from build123d import *

# Parameters (mm, degrees)
EXTRUDE_THIN1_DEPTH = 12.7
CUT_EXTRUDE1_REACH  = 74.956
SKETCH2_R           = 2.25
CUT_EXTRUDE2_REACH  = 74.956
SKETCH6_R           = 1.5


with BuildPart() as part:
    # Sketch1 → Extrude-Thin1 (new body)
    with BuildSketch(Plane.XY):
        Polygon((0, 0), (0, 50.8), (50.8, 50.8), (50.8, 47.625), (3.175, 47.625), (3.175, 0), align=None)
    extrude(amount=EXTRUDE_THIN1_DEPTH)

    # Sketch2 → Cut-Extrude1 (cut, up to next)
    with BuildSketch(Plane.ZY, mode=Mode.PRIVATE) as cut_extrude1_sk1:
        with Locations((6.35, 12.7)):
            Circle(SKETCH2_R)
    cut_extrude1_tool1 = extrude(cut_extrude1_sk1.sketch, amount=-CUT_EXTRUDE1_REACH, mode=Mode.PRIVATE) & part.part
    # Sketch2 → Cut-Extrude1 (cut, up to next)
    with BuildSketch(Plane.ZY, mode=Mode.PRIVATE) as cut_extrude1_sk2:
        with Locations((6.35, 25.4)):
            Circle(SKETCH2_R)
    cut_extrude1_tool2 = extrude(cut_extrude1_sk2.sketch, amount=-CUT_EXTRUDE1_REACH, mode=Mode.PRIVATE) & part.part
    add(cut_extrude1_tool1.solids().sort_by_distance((0, 12.7, 6.35))[0], mode=Mode.SUBTRACT)
    add(cut_extrude1_tool2.solids().sort_by_distance((0, 25.4, 6.35))[0], mode=Mode.SUBTRACT)

    # Sketch6 → Cut-Extrude2 (cut, up to next)
    with BuildSketch(Plane(origin=(0, 50.8, 0), x_dir=(1, 0, 0), z_dir=(0, 1, 0)), mode=Mode.PRIVATE) as cut_extrude2_sk1:
        with Locations(Location((24.25, -6.35, 0), (0, 0, 270))):
            Circle(SKETCH6_R)
    cut_extrude2_tool1 = extrude(cut_extrude2_sk1.sketch, amount=-CUT_EXTRUDE2_REACH, mode=Mode.PRIVATE) & part.part
    # Sketch6 → Cut-Extrude2 (cut, up to next)
    with BuildSketch(Plane(origin=(0, 50.8, 0), x_dir=(1, 0, 0), z_dir=(0, 1, 0)), mode=Mode.PRIVATE) as cut_extrude2_sk2:
        with Locations(Location((39.25, -6.35, 0), (0, 0, 270))):
            Circle(SKETCH6_R)
    cut_extrude2_tool2 = extrude(cut_extrude2_sk2.sketch, amount=-CUT_EXTRUDE2_REACH, mode=Mode.PRIVATE) & part.part
    add(cut_extrude2_tool1.solids().sort_by_distance((24.25, 50.8, 6.35))[0], mode=Mode.SUBTRACT)
    add(cut_extrude2_tool2.solids().sort_by_distance((39.25, 50.8, 6.35))[0], mode=Mode.SUBTRACT)


solid = part.part
Geometry check sheet. Reference: the model listing, model coordinates, mm. A direction names the side the tool comes from. Round coordinates to 2 decimals unless told otherwise and drop trailing zeros. Loops run counter-clockwise (first coordinate to the right, second up) from the corner with the lowest first, then second, coordinate; pieces in that order, holes last. Notation, with made-up numbers: (83, -30) - (98, -30) arc R21 cw to (98, -15) - close; hole circle Ø5 at (44, 53). An arc over 180 degrees is marked (long way). Answer as CSV lines item,"result".
(1) Cross-section at C-C, the plane z = 6.25. Enter the section's corners in (x, y) (3 decimals).
Output values:
outline,"(0, 0) - (3.175, 0) - (3.175, 10.452) - (0, 10.452) - close; (0, 14.948) - (3.175, 14.948) - (3.175, 23.152) - (0, 23.152) - close; (0, 27.648) - (3.175, 27.648) - (3.175, 47.625) - (22.753, 47.625) - (22.753, 50.8) - (0, 50.8) - close; (25.747, 47.625) - (37.753, 47.625) - (37.753, 50.8) - (25.747, 50.8) - close; (40.747, 47.625) - (50.8, 47.625) - (50.8, 50.8) - (40.747, 50.8) - close"
(2) Depth check by flat-ended pin: pin 1 Ø4 at (y, z) = (25.4, 6.35) entering from +X; pin 2 Ø1.5 at (y, z) = (36.5, 3) entering from +X (3 decimals); pin 3 Ø6.5 at (x, z) = (19.5, 8.5) entering from -Y (3 decimals). Enter the tip coordinate at first touch or a pass-through.
Output values:
pin 1,"passes through"
pin 2,"stops at x = 3.175"
pin 3,"stops at y = 47.625"
(3) Material ranges on line 1 along X through (y, z) = (49.2, 6.35); line 2 along Y through (x, z) = (1.3, 6.35); line 3 along Y through (x, z) = (31, 4.25) (3 decimals), recorded low to high.
Output values:
line 1,"x = 0 to 22.75, 25.75 to 37.75, 40.75 to 50.8"
line 2,"y = 0 to 10.45, 14.95 to 23.15, 27.65 to 50.8"
line 3,"y = 47.625 to 50.8"
(4) Cross-section at B-B, the plane x = 24.25. Enter the section's corners in (y, z) (3 decimals), and give its area (3 significant figures).
Output values:
outline,"(47.625, 0) - (50.8, 0) - (50.8, 4.85) - (47.625, 4.85) - close; (47.625, 7.85) - (50.8, 7.85) - (50.8, 12.7) - (47.625, 12.7) - close"
area,"30.8 mm²"
(5) Cross-section at A-A, the plane y = 12.7. Enter the section's corners in (x, z) (3 decimals).
Output values:
outline,"(0, 0) - (3.175, 0) - (3.175, 4.1) - (0, 4.1) - close; (0, 8.6) - (3.175, 8.6) - (3.175, 12.7) - (0, 12.7) - close"
(6) Set-up check for faces 1 (the face through (1.57, 27.63, 6.06)), 2 (the face through (3.175, 24, 9)): record each of +Z, -Z, +X, -X, +Y, -Y from which the full face is reachable in a straight line by a thin tool's end or side.
Output values:
face 1,"+X, -X"
face 2,"+Z, -Z, +X, -Y"
(7) Release check for a two-part mould opening along Z. For faces 3 (the face through (25.737, 49.235, 6.155)), 4 (the face through (2, 0, 6)), 5 (the face through (14, 48, 12.7)), 6 (the face through (1.565, 10.504, 5.862)) record: released by +Z, released by -Z, zero draft, split by the parting line, or undercut.
Output values:
face 3,"undercut"
face 4,"zero draft"
face 5,"released by +Z"
face 6,"undercut"
(8) Cross-section at D-D, the plane y = 33. Enter the section's corners in (x, z) (3 decimals).
Output values:
outline,"(0, 0) - (3.175, 0) - (3.175, 12.7) - (0, 12.7) - close"
